Read the model definition and answer for the solid it produces. Units are mm, in the model's axes. Face numbers are marked on the shaded views. A direction names the side the tool comes from. Give positions to 0.01 mm unless a question says otherwise; leave off trailing zeros. Write each loop counter-clockwise with the first axis right and the second up, starting at its lowest first coordinate (ties: lowest second). Pieces come first, ordered by that corner, then holes. Notation, with made-up numbers: (29, -12) -> (87, -12) arc R28 ccw to (87, 19) -> close; hole circle Ø10 at (39.5, -33). An arc over 180 degrees is marked (long way). Use a Markdown table: item, result.
from build123d import *

# Parameters (mm, degrees)
SKETCH1_W           = 30
SKETCH1_H           = 30
SKETCH1_R           = 3.1
BOSS_EXTRUDE1_DEPTH = 13
SKETCH2_R           = 9
CUT_EXTRUDE1_DEPTH  = 8
FILLET1_R           = 2


with BuildPart() as part:
    # Sketch1 → Boss-Extrude1 (new body)
    with BuildSketch(Plane.XY):
        Rectangle(SKETCH1_W, SKETCH1_H)
        Circle(SKETCH1_R, mode=Mode.SUBTRACT)
    extrude(amount=BOSS_EXTRUDE1_DEPTH)

    # Sketch2 → Cut-Extrude1 (cut)
    with BuildSketch(Plane.XY.offset(13)):
        Circle(SKETCH2_R)
    extrude(amount=-CUT_EXTRUDE1_DEPTH, mode=Mode.SUBTRACT)

    # Fillet1
    fillet1_edges = [part.edges().sort_by_distance(p)[0] for p in [
        (15, -15, 6.5),
        (-15, -15, 6.5),
        (-15, 15, 6.5),
        (15, 15, 6.5),
    ]]
    fillet(fillet1_edges, radius=FILLET1_R)


solid = part.part
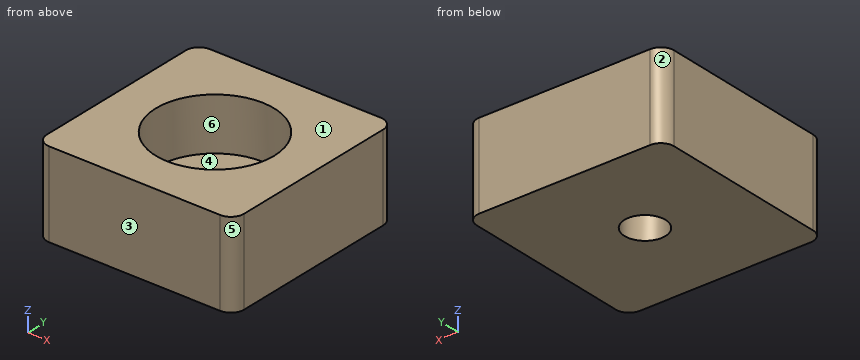
Item 1: This flat-tipped pin is pushed along its axis until it touches: P1, Ø8, axis at x = 0, y = 0, coming from the -Z side. Where does it stop, or does it pass through?
Return value:
| item | result |
|---|---|
| P1 | z = 0 |
Item 2: A cutting plane is placed at D-D (z = 8.5). Give the vertices of the cut face in (x, y).
Return value:
| item | result |
|---|---|
| outline | (-15, -13) arc R2 ccw to (-13, -15) -> (13, -15) arc R2 ccw to (15, -13) -> (15, 13) arc R2 ccw to (13, 15) -> (-13, 15) arc R2 ccw to (-15, 13) -> close; hole circle Ø18 at (0, 0) |
Item 3: A cutting plane is placed at C-C (z = 3). Give the vertices of the cut face in (x, y).
Return value:
| item | result |
|---|---|
| outline | (-15, -13) arc R2 ccw to (-13, -15) -> (13, -15) arc R2 ccw to (15, -13) -> (15, 13) arc R2 ccw to (13, 15) -> (-13, 15) arc R2 ccw to (-15, 13) -> close; hole circle Ø6.2 at (0, 0) |
Item 4: A tool of negligible diameter and unlimited length cuts with its end or side. For the marked faces 5 and 6, from which of +Z, -Z, +X, -X, +Y, -Y can it reach the whole face along a straight path? Write none if from no direction.
Return value:
| item | result |
|---|---|
| face 5 | +Z, -Z, +X, -Y |
| face 6 | +Z |
Item 5: For a pull along Y with two mould halves and no side action, classify the marked faces 1, 2, 3 and 4 as +Y half, -Y half, draft (parallel to the pull), parting line (faces both ways), or undercut.
Return value:
| item | result |
|---|---|
| face 1 | draft |
| face 2 | +Y half |
| face 3 | -Y half |
| face 4 | undercut |
Item 6: A cutting plane is placed at A-A (x = 0). Give the vertices of the cut face in (y, z), then the cut area to 3 significant figures.
Return value:
| item | result |
|---|---|
| outline | (-15, 0) -> (-3.1, 0) -> (-3.1, 5) -> (-9, 5) -> (-9, 13) -> (-15, 13) -> close; (3.1, 0) -> (15, 0) -> (15, 13) -> (9, 13) -> (9, 5) -> (3.1, 5) -> close |
| area | 215 mm^2 |
Item 7: Straight lines are drawn through the part: line 1 along X through (y, z) = (0, 2.6); line 2 along Y through (x, z) = (0, 8.25). For each, find the intervals that lie inside material, in ascending order. Write a range as [from, to].
Return value:
| item | result |
|---|---|
| line 1 | [-15, -3.1], [3.1, 15] |
| line 2 | [-15, -9], [9, 15] |
